```python
from build123d import *

# Parameters (mm, degrees)
F0_W      = 19.05
F0_H      = 76.2
F1_DEPTH  = 5
F2_W      = 3.5
F2_H      = 7.5
F2_W_2    = 6
F2_H_2    = 5
F3_DEPTH  = 5
F4_R      = 3.175
F5_DEPTH  = 5
F3_FACE_W = 3.5
F3_FACE_H = 7.5
F6_DEPTH  = 1.5


with BuildPart() as f1:
    # F0 (on Top) → F1 (new body)
    with BuildSketch(Plane.XY):
        Rectangle(F0_W, F0_H)
    extrude(amount=F1_DEPTH)

    # F2 (on face) → F3 (join)
    with BuildSketch(Plane.XY.offset(5)):
        with Locations((0, 34.35)):
            Rectangle(F2_W, F2_H)
        with Locations((-6.525, -35.6)):
            Rectangle(F2_W_2, F2_H_2)
        with Locations((6.525, -35.6)):
            Rectangle(F2_W_2, F2_H_2)
    extrude(amount=F3_DEPTH)

    # F4 (on face) → F5 (cut)
    with BuildSketch(Plane.XY.offset(5)):
        with Locations((0, 16.04)):
            Circle(F4_R)
        with Locations((0, -16.04)):
            Circle(F4_R)
    extrude(amount=-F5_DEPTH, mode=Mode.SUBTRACT)

    # F3_face (on face) → F6 (cut)
    with BuildSketch(Plane(origin=(0, 34.35, 10), x_dir=(1, 0, 0), z_dir=(0, 0, 1))):
        Rectangle(F3_FACE_W, F3_FACE_H)
    extrude(amount=-F6_DEPTH, mode=Mode.SUBTRACT)


solid = f1.part
```
Model file for the job. Use its own axes, mm. A direction names the side the tool comes from. Give positions to 0.01 mm unless a question says otherwise; leave off trailing zeros. Write each loop counter-clockwise with the first axis right and the second up, starting at its lowest first coordinate (ties: lowest second). Pieces come first, ordered by that corner, then holes. Notation, with made-up numbers: M 10,-3.75 L 32,-3.75 A25 cw 32,22.25 Z; hole C 46,-29.5 d6. An arc over 180 degrees is marked long. Use a Markdown table: item, result.
1) Drill centre lines: line 1 (Y direction, x = 0, z = 2.1) (3 decimals); line 2 (Z direction, x = 6.5, y = -20); line 3 (Y direction, x = 6.25, z = 9.75). Where is each one in solid material? Low to high. Write a range as from..to.
Responses:
| item | result |
|---|---|
| line 1 | y = -38.1..-19.215, -12.865..12.865, 19.215..38.1 |
| line 2 | z = 0..5 |
| line 3 | y = -38.1..-33.1 |
2) Pull direction Y, two halves, no side cores. Call faces 6 (the flat face through (0, 1, 0)), 7 (the flat face through (0, -38.1, 4)), 8 (the cylindrical face through (3, -15, 3)): +Y half, -Y half, draft (parallel to the pull), parting line (faces both ways), or undercut.
Responses:
| item | result |
|---|---|
| face 6 | draft |
| face 7 | -Y half |
| face 8 | undercut |
3) Cut at D-D (y = -3.5). List the corners of the cut face in (x, z) (3 decimals), and give its area (4 significant figures).
Responses:
| item | result |
|---|---|
| outline | M -9.525,0 L 9.525,0 L 9.525,5 L -9.525,5 Z |
| area | 95.25 mm2 |
4) Tool access for faces 1 (the flat face through (0, 30.6, 7)), 2 (the flat face through (-7, -33.1, 7)), 3 (the flat face through (-1.75, 34, 7)), 4 (the flat face through (1.75, 34, 7)), 5 (the flat face through (-3.525, -36, 7)): list every direction of +Z, -Z, +X, -X, +Y, -Y with a clear straight run to the whole face (end or side of a thin tool).
Responses:
| item | result |
|---|---|
| face 1 | +Z, +X, -X, -Y |
| face 2 | +Z, +X, -X, +Y |
| face 3 | +Z, -X, +Y, -Y |
| face 4 | +Z, +X, +Y, -Y |
| face 5 | +Z, +Y, -Y |
5) Cut at A-A (y = -16.04). List the corners of the cut face in (x, z) (3 decimals), and give its area (3 significant figures).
Responses:
| item | result |
|---|---|
| outline | M -9.525,0 L -3.175,0 L -3.175,5 L -9.525,5 Z; M 3.175,0 L 9.525,0 L 9.525,5 L 3.175,5 Z |
| area | 63.5 mm2 |
6) Pin check, flat tips, straight feed: pin 1 (2 mm diameter, centred on x = -3, z = 7.5, fed in from -Y); pin 2 (5.5 mm diameter, centred on x = -4, y = -11, fed in from +Z); pin 3 (2.5 mm diameter, centred on x = -5, z = 7.5, fed in from +Y); pin 4 (1.8 mm diameter, centred on y = 35.5, z = 7, fed in from +X). Stop position of each tip, or through.
Responses:
| item | result |
|---|---|
| pin 1 | stops at y = -38.1 |
| pin 2 | stops at z = 5 |
| pin 3 | stops at y = -33.1 |
| pin 4 | stops at x = 1.75 |
7) Cut at C-C (z = 2). List the corners of the cut face in (x, y) (3 decimals).
Responses:
| item | result |
|---|---|
| outline | M -9.525,-38.1 L 9.525,-38.1 L 9.525,38.1 L -9.525,38.1 Z; hole C 0,-16.04 d6.35; hole C 0,16.04 d6.35 |
8) Cut at B-B (z = 6.75). List the corners of the cut face in (x, y) (3 decimals), and give its area (4 significant figures).
Responses:
| item | result |
|---|---|
| outline | M -9.525,-38.1 L -3.525,-38.1 L -3.525,-33.1 L -9.525,-33.1 Z; M -1.75,30.6 L 1.75,30.6 L 1.75,38.1 L -1.75,38.1 Z; M 3.525,-38.1 L 9.525,-38.1 L 9.525,-33.1 L 3.525,-33.1 Z |
| area | 86.25 mm2 |
